For this review, take the finished solid that the model builds, in its own axes (mm). A direction names the side the tool comes from. Give positions to 0.01 mm unless a question says otherwise; leave off trailing zeros. Write each loop counter-clockwise with the first axis right and the second up, starting at its lowest first coordinate (ties: lowest second). Pieces come first, ordered by that corner, then holes.
from build123d import *

# Parameters (mm, degrees)
BASE_R              = 3.05
BOSS_EXTRUDE1_DEPTH = 2
BOSS_EXTRUDE2_START = 2
BASE_3_R            = 30
BASE_3_R_2          = 26.5
BASE_3_R_3          = 3.05
BOSS_EXTRUDE2_DEPTH = 3
FILLET1_R           = 2
CHAMFER1_SIZE       = 1
BASE_4_R            = 3.05
CUT_EXTRUDE1_DEPTH  = 3.5


with BuildPart() as part:
    # Base → Boss-Extrude1 (new body)
    # profile 1 of 8: a face of its own
    with BuildSketch(Plane(origin=(0, 0, 0), x_dir=(1, 0, 0), z_dir=(0, 1, 0))):
        with BuildLine():
            Line((-23.037821007, -30.108888819), (-30.108888819, -23.037821007))
            Line((-30.108888819, -23.037821007), (-35.765743068, -28.694675256))
            ThreePointArc((-35.765743068, -28.694675256), (-35.765743068, -35.765743068), (-28.694675256, -35.765743068))
            Line((-28.694675256, -35.765743068), (-23.037821007, -30.108888819))
        make_face()
        with Locations((-32.230209162, -32.230209162)):
            Circle(BASE_R, mode=Mode.SUBTRACT)
    # profile 2 of 8: a face of its own
    with BuildSketch(Plane(origin=(0, 0, 0), x_dir=(1, 0, 0), z_dir=(0, 1, 0))):
        with BuildLine():
            Line((35.765743068, -28.694675256), (30.108888819, -23.037821007))
            Line((30.108888819, -23.037821007), (23.037821007, -30.108888819))
            Line((23.037821007, -30.108888819), (28.694675256, -35.765743068))
            ThreePointArc((28.694675256, -35.765743068), (35.765743068, -35.765743068), (35.765743068, -28.694675256))
        make_face()
        with Locations((32.230209162, -32.230209162)):
            Circle(BASE_R, mode=Mode.SUBTRACT)
    # profile 3 of 8: a face of its own
    with BuildSketch(Plane(origin=(0, 0, 0), x_dir=(1, 0, 0), z_dir=(0, 1, 0))):
        with BuildLine():
            Line((28.694675256, 35.765743068), (23.037821007, 30.108888819))
            Line((23.037821007, 30.108888819), (30.108888819, 23.037821007))
            Line((30.108888819, 23.037821007), (35.765743068, 28.694675256))
            ThreePointArc((35.765743068, 28.694675256), (35.765743068, 35.765743068), (28.694675256, 35.765743068))
        make_face()
        with Locations((32.230209162, 32.230209162)):
            Circle(BASE_R, mode=Mode.SUBTRACT)
    # profile 4 of 8: a face of its own
    with BuildSketch(Plane(origin=(0, 0, 0), x_dir=(1, 0, 0), z_dir=(0, 1, 0))):
        with BuildLine():
            Line((-23.037821007, 30.108888819), (-28.694675256, 35.765743068))
            ThreePointArc((-28.694675256, 35.765743068), (-35.765743068, 35.765743068), (-35.765743068, 28.694675256))
            Line((-35.765743068, 28.694675256), (-30.108888819, 23.037821007))
            Line((-30.108888819, 23.037821007), (-23.037821007, 30.108888819))
        make_face()
        with Locations((-32.230209162, 32.230209162)):
            Circle(BASE_R, mode=Mode.SUBTRACT)
    # profile 5 of 8: a face of its own
    with BuildSketch(Plane(origin=(0, 0, 0), x_dir=(1, 0, 0), z_dir=(0, 1, 0))):
        with Locations((32.230209162, 32.230209162)):
            Circle(BASE_R)
    # profile 6 of 8: a face of its own
    with BuildSketch(Plane(origin=(0, 0, 0), x_dir=(1, 0, 0), z_dir=(0, 1, 0))):
        with Locations((-32.230209162, 32.230209162)):
            Circle(BASE_R)
    # profile 7 of 8: a face of its own
    with BuildSketch(Plane(origin=(0, 0, 0), x_dir=(1, 0, 0), z_dir=(0, 1, 0))):
        with Locations((-32.230209162, -32.230209162)):
            Circle(BASE_R)
    # profile 8 of 8: a face of its own
    with BuildSketch(Plane(origin=(0, 0, 0), x_dir=(1, 0, 0), z_dir=(0, 1, 0))):
        with Locations((32.230209162, -32.230209162)):
            Circle(BASE_R)
    extrude(amount=BOSS_EXTRUDE1_DEPTH)

    # Base<3> → Boss-Extrude2 (add)
    # profile 1 of 13: a face of its own
    with BuildSketch(Plane(origin=(0, 0, 0), x_dir=(1, 0, 0), z_dir=(0, 1, 0)).offset(BOSS_EXTRUDE2_START)):
        Circle(BASE_3_R)
        with Locations(Location((0, 0, 0), (0, 0, 270))):
            Circle(BASE_3_R_2, mode=Mode.SUBTRACT)
    # profile 2 of 13: a face of its own
    with BuildSketch(Plane(origin=(0, 0, 0), x_dir=(1, 0, 0), z_dir=(0, 1, 0)).offset(BOSS_EXTRUDE2_START)):
        with BuildLine():
            ThreePointArc((-17.380966757, -24.452034569), (-21.213203436, -21.213203436), (-24.452034569, -17.380966757))
            Line((-24.452034569, -17.380966757), (-30.108888819, -23.037821007))
            Line((-30.108888819, -23.037821007), (-23.037821007, -30.108888819))
            Line((-23.037821007, -30.108888819), (-17.380966757, -24.452034569))
        make_face()
    # profile 3 of 13: a face of its own
    with BuildSketch(Plane(origin=(0, 0, 0), x_dir=(1, 0, 0), z_dir=(0, 1, 0)).offset(BOSS_EXTRUDE2_START)):
        with BuildLine():
            Line((-23.037821007, -30.108888819), (-30.108888819, -23.037821007))
            Line((-30.108888819, -23.037821007), (-35.765743068, -28.694675256))
            ThreePointArc((-35.765743068, -28.694675256), (-35.765743068, -35.765743068), (-28.694675256, -35.765743068))
            Line((-28.694675256, -35.765743068), (-23.037821007, -30.108888819))
        make_face()
        with Locations((-32.230209162, -32.230209162)):
            Circle(BASE_3_R_3, mode=Mode.SUBTRACT)
    # profile 4 of 13: a face of its own
    with BuildSketch(Plane(origin=(0, 0, 0), x_dir=(1, 0, 0), z_dir=(0, 1, 0)).offset(BOSS_EXTRUDE2_START)):
        with BuildLine():
            Line((30.108888819, -23.037821007), (24.452034569, -17.380966757))
            ThreePointArc((24.452034569, -17.380966757), (21.213203436, -21.213203436), (17.380966757, -24.452034569))
            Line((17.380966757, -24.452034569), (23.037821007, -30.108888819))
            Line((23.037821007, -30.108888819), (30.108888819, -23.037821007))
        make_face()
    # profile 5 of 13: a face of its own
    with BuildSketch(Plane(origin=(0, 0, 0), x_dir=(1, 0, 0), z_dir=(0, 1, 0)).offset(BOSS_EXTRUDE2_START)):
        with BuildLine():
            Line((35.765743068, -28.694675256), (30.108888819, -23.037821007))
            Line((30.108888819, -23.037821007), (23.037821007, -30.108888819))
            Line((23.037821007, -30.108888819), (28.694675256, -35.765743068))
            ThreePointArc((28.694675256, -35.765743068), (35.765743068, -35.765743068), (35.765743068, -28.694675256))
        make_face()
        with Locations((32.230209162, -32.230209162)):
            Circle(BASE_3_R_3, mode=Mode.SUBTRACT)
    # profile 6 of 13: a face of its own
    with BuildSketch(Plane(origin=(0, 0, 0), x_dir=(1, 0, 0), z_dir=(0, 1, 0)).offset(BOSS_EXTRUDE2_START)):
        with BuildLine():
            Line((23.037821007, 30.108888819), (17.380966757, 24.452034569))
            ThreePointArc((17.380966757, 24.452034569), (21.213203436, 21.213203436), (24.452034569, 17.380966757))
            Line((24.452034569, 17.380966757), (30.108888819, 23.037821007))
            Line((30.108888819, 23.037821007), (23.037821007, 30.108888819))
        make_face()
    # profile 7 of 13: a face of its own
    with BuildSketch(Plane(origin=(0, 0, 0), x_dir=(1, 0, 0), z_dir=(0, 1, 0)).offset(BOSS_EXTRUDE2_START)):
        with BuildLine():
            Line((28.694675256, 35.765743068), (23.037821007, 30.108888819))
            Line((23.037821007, 30.108888819), (30.108888819, 23.037821007))
            Line((30.108888819, 23.037821007), (35.765743068, 28.694675256))
            ThreePointArc((35.765743068, 28.694675256), (35.765743068, 35.765743068), (28.694675256, 35.765743068))
        make_face()
        with Locations((32.230209162, 32.230209162)):
            Circle(BASE_3_R_3, mode=Mode.SUBTRACT)
    # profile 8 of 13: a face of its own
    with BuildSketch(Plane(origin=(0, 0, 0), x_dir=(1, 0, 0), z_dir=(0, 1, 0)).offset(BOSS_EXTRUDE2_START)):
        with BuildLine():
            Line((-17.380966757, 24.452034569), (-23.037821007, 30.108888819))
            Line((-23.037821007, 30.108888819), (-30.108888819, 23.037821007))
            Line((-30.108888819, 23.037821007), (-24.452034569, 17.380966757))
            ThreePointArc((-24.452034569, 17.380966757), (-21.213203436, 21.213203436), (-17.380966757, 24.452034569))
        make_face()
    # profile 9 of 13: a face of its own
    with BuildSketch(Plane(origin=(0, 0, 0), x_dir=(1, 0, 0), z_dir=(0, 1, 0)).offset(BOSS_EXTRUDE2_START)):
        with BuildLine():
            Line((-23.037821007, 30.108888819), (-28.694675256, 35.765743068))
            ThreePointArc((-28.694675256, 35.765743068), (-35.765743068, 35.765743068), (-35.765743068, 28.694675256))
            Line((-35.765743068, 28.694675256), (-30.108888819, 23.037821007))
            Line((-30.108888819, 23.037821007), (-23.037821007, 30.108888819))
        make_face()
        with Locations((-32.230209162, 32.230209162)):
            Circle(BASE_3_R_3, mode=Mode.SUBTRACT)
    # profile 10 of 13: a face of its own
    with BuildSketch(Plane(origin=(0, 0, 0), x_dir=(1, 0, 0), z_dir=(0, 1, 0)).offset(BOSS_EXTRUDE2_START)):
        with Locations((-32.230209162, 32.230209162)):
            Circle(BASE_3_R_3)
    # profile 11 of 13: a face of its own
    with BuildSketch(Plane(origin=(0, 0, 0), x_dir=(1, 0, 0), z_dir=(0, 1, 0)).offset(BOSS_EXTRUDE2_START)):
        with Locations((-32.230209162, -32.230209162)):
            Circle(BASE_3_R_3)
    # profile 12 of 13: a face of its own
    with BuildSketch(Plane(origin=(0, 0, 0), x_dir=(1, 0, 0), z_dir=(0, 1, 0)).offset(BOSS_EXTRUDE2_START)):
        with Locations((32.230209162, -32.230209162)):
            Circle(BASE_3_R_3)
    # profile 13 of 13: a face of its own
    with BuildSketch(Plane(origin=(0, 0, 0), x_dir=(1, 0, 0), z_dir=(0, 1, 0)).offset(BOSS_EXTRUDE2_START)):
        with Locations((32.230209162, 32.230209162)):
            Circle(BASE_3_R_3)
    extrude(amount=BOSS_EXTRUDE2_DEPTH)

    # Fillet1
    fillet1_edges = [part.edges().sort_by_distance(p)[0] for p in [
        (24.452034569, 3.5, 17.380966757),
        (-17.380966757, 3.5, -24.452034569),
        (24.452034569, 3.5, -17.380966757),
        (-17.380966757, 3.5, 24.452034569),
        (17.380966757, 3.5, -24.452034569),
        (-24.452034569, 3.5, 17.380966757),
        (17.380966757, 3.5, 24.452034569),
        (-24.452034569, 3.5, -17.380966757),
        (-26.573354913, 2, 26.573354913),
        (-26.573354913, 2, -26.573354913),
        (26.573354913, 2, 26.573354913),
        (26.573354913, 2, -26.573354913),
    ]]
    fillet(fillet1_edges, radius=FILLET1_R - 0.0001)  # a hair under: the kernel refuses the full size

    # Chamfer1
    chamfer1_edges = [part.edges().sort_by_distance(p)[0] for p in [
        (23.619243451, 5, 30.690311263),
        (0, 5, 30),
        (-23.619243451, 5, 30.690311263),
        (-30.690311263, 5, 23.619243451),
        (-30, 5, 0),
        (-30.690311263, 5, -23.619243451),
        (-23.619243451, 5, -30.690311263),
        (0, 5, -30),
        (30.690311263, 5, -23.619243451),
        (30, 5, 0),
        (30.690311263, 5, 23.619243451),
        (23.619243451, 5, -30.690311263),
        (-29.694695967, 1.414242852, 22.623628155),
        (-22.623628155, 1.414242852, 29.694695967),
        (-22.623628155, 1.414242852, -29.694695967),
        (-29.694695967, 1.414242852, -22.623628155),
        (22.623628155, 1.414242852, 29.694695967),
        (29.694695967, 1.414242852, 22.623628155),
        (29.694695967, 1.414242852, -22.623628155),
        (22.623628155, 1.414242852, -29.694695967),
        (17.349741935, 2, 25.041267842),
        (17.349741935, 5, 25.041267842),
        (-17.349741935, 2, 25.041267842),
        (-17.349741935, 5, 25.041267842),
        (-25.041267842, 2, 17.349741935),
        (-25.041267842, 5, 17.349741935),
        (-25.041267842, 2, -17.349741935),
        (-25.041267842, 5, -17.349741935),
        (-17.349741935, 2, -25.041267842),
        (-17.349741935, 5, -25.041267842),
        (25.041267842, 2, -17.349741935),
        (25.041267842, 5, -17.349741935),
        (25.041267842, 2, 17.349741935),
        (25.041267842, 5, 17.349741935),
        (17.349741935, 2, -25.041267842),
        (17.349741935, 5, -25.041267842),
        (0, 2, -26.5),
        (35.765743068, 5, 35.765743068),
        (35.765743068, 5, -35.765743068),
        (-35.765743068, 5, -35.765743068),
        (-35.765743068, 5, 35.765743068),
        (-20.083744901, 2, -27.154812712),
        (0, 2, -30),
        (20.083744901, 2, -27.154812712),
        (27.154812712, 2, -20.083744901),
        (30, 2, 0),
        (27.154812712, 2, 20.083744901),
        (20.083744901, 2, 27.154812712),
        (0, 2, 30),
        (-20.083744901, 2, 27.154812712),
        (-27.154812712, 2, 20.083744901),
        (-30, 2, 0),
        (-27.154812712, 2, -20.083744901),
    ]]
    chamfer(chamfer1_edges, length=CHAMFER1_SIZE)

    # Base<4> → Cut-Extrude1 (cut)
    with BuildSketch(Plane(origin=(0, 0, 0), x_dir=(1, 0, 0), z_dir=(0, 1, 0))):
        with Locations(Location((32.230209162, -32.230209162, 0), (0, 0, 270))):
            Circle(BASE_4_R)
        with Locations(Location((-32.230209162, -32.230209162, 0), (0, 0, 270))):
            Circle(BASE_4_R)
        with Locations(Location((-32.230209162, 32.230209162, 0), (0, 0, 270))):
            Circle(BASE_4_R)
        with Locations(Location((32.230209162, 32.230209162, 0), (0, 0, 270))):
            Circle(BASE_4_R)
    extrude(amount=CUT_EXTRUDE1_DEPTH, mode=Mode.SUBTRACT)


solid = part.part
(1) Clearance check with flat-ended pins moving along their axes: pin 1 Ø3 at (x, z) = (32.5, -33.5) entering from -Y; pin 2 Ø2 at (x, y) = (23, 4) entering from +Z; pin 3 Ø3 at (x, y) = (-23.5, 3) entering from -Z. State where each tip first meets the part, or that it passes through.
(2) We need section B-B (x = 0). Write out the cut boundary in (y, z).
(3) Tool access review of faces 1 (the flat face through (26.818, 2.493, 20.464)), 2 (the flat face through (31.75, 2.42, -24.68)), 3 (the flat face through (-24.68, 2.42, -31.75)), 4 (the flat face through (-32, 3.5, 32)): name each direction out of +Z, -Z, +X, -X, +Y, -Y from which nothing blocks a thin tool from reaching the whole face with its end or side.
(4) We need section A-A (z = 0). Write out the cut boundary in (x, y), and give its area (3 significant figures).
(5) For L1, parallel to Z at x = 31.5, y = 2.7; L2, parallel to Z at x = 27.5, y = 3.7; L3, parallel to X at y = 3.4, z = 1, list the stretches that pass through material, from the lowest coordinate up.
(6) The part is to be moulded in two halves that separate along Z. For faces 5 (the conical face through (23.24, 1.7, 29.44)), 6 (the flat face through (30.271, 4.493, -23.897)), 7 (the conical face through (23.24, 1.7, -29.44)), say which applies: +Z half, -Z half, draft (parallel to the pull), parting line (faces both ways), or undercut.
The answers:
1. pin 1: stops at y = 3.5
1. pin 2: stops at z = 31.07
1. pin 3: stops at z = -32.07
2. outline: (2, -29) - (3, -30) - (4, -30) - (5, -29) - (5, -26.5) - (3, -26.5) - (2, -27.5) - close; (2, 27.5) - (3, 26.5) - (5, 26.5) - (5, 29) - (4, 30) - (3, 30) - (2, 29) - close
3. face 1: +X, -Y
3. face 2: +X, +Y, -Y
3. face 3: -Z, +Y, -Y
3. face 4: -Y
4. outline: (-30, 3) - (-29, 2) - (-27.5, 2) - (-26.5, 3) - (-26.5, 5) - (-29, 5) - (-30, 4) - close; (26.5, 3) - (27.5, 2) - (29, 2) - (30, 3) - (30, 4) - (29, 5) - (26.5, 5) - close
4. area: 18.0 mm2
5. L1: z = -37.18 to -35.19, -29.27 to -24.43, 24.43 to 29.27, 35.19 to 37.18
5. L2: z = -34.57 to -20.43, -11.99 to 11.99, 20.43 to 34.57
5. L3: x = -29.98 to -26.48, 26.48 to 29.98
6. face 5: +Z half
6. face 6: undercut
6. face 7: -Z half
